The model under review builds one solid part; all positions refer to its coordinate system, in mm. A direction names the side the tool comes from. Coordinates: 2 decimals unless noted, no trailing zeros. Write each loop counter-clockwise with the first axis right and the second up, starting at its lowest first coordinate (ties: lowest second). Pieces come first, ordered by that corner, then holes. Notation, with made-up numbers: (88.5, -5) - (133.5, -5) arc R15 cw to (133.5, 18) - close; hole circle Ø10 at (-21.5, 53). An arc over 180 degrees is marked (long way). Use one line per item in the form item = value. Start each with the question number.
```python
from build123d import *

# Parameters (mm, degrees)
SKETCH_W        = 95
SKETCH_H        = 27
PAD_DEPTH       = 2
SKETCH001_R     = 1.3
POCKET_DEPTH    = 2
FILLET_R        = 3
SKETCH002_W     = 9.2
SKETCH002_H     = 11.4
POCKET001_DEPTH = 2
SKETCH003_W     = 13.2
SKETCH003_H     = 11.4
SKETCH003_W_2   = 18.2
SKETCH003_H_2   = 11.5
POCKET002_DEPTH = 2


with BuildPart() as part:
    # Sketch → Pad (new body)
    with BuildSketch(Plane.XY):
        Rectangle(SKETCH_W, SKETCH_H)
    extrude(amount=PAD_DEPTH)

    # Sketch001 (on Face6 of Pad) → Pocket (cut)
    with BuildSketch(Plane.XY.offset(2)):
        with Locations((-44.5, 10.5)):
            Circle(SKETCH001_R)
        with Locations((44.5, 10.5)):
            Circle(SKETCH001_R)
        with Locations((44.5, -10.5)):
            Circle(SKETCH001_R)
        with Locations((-44.5, -10.5)):
            Circle(SKETCH001_R)
    extrude(amount=-POCKET_DEPTH, mode=Mode.SUBTRACT)

    # Fillet
    fillet_edges = [part.edges().sort_by_distance(p)[0] for p in [
        (-47.5, -13.5, 1),
        (47.5, -13.5, 1),
        (47.5, 13.5, 1),
        (-47.5, 13.5, 1),
    ]]
    fillet(fillet_edges, radius=FILLET_R)

    # Sketch002 (on Face5 of Fillet) → Pocket001 (cut)
    with BuildSketch(Plane.XY.offset(2)):
        with Locations((31.3, 1.1)):
            Rectangle(SKETCH002_W, SKETCH002_H)
    extrude(amount=-POCKET001_DEPTH, mode=Mode.SUBTRACT)

    # Sketch003 (on Face5 of Pocket001) → Pocket002 (cut)
    with BuildSketch(Plane.XY.offset(2)):
        with Locations((4, 1.1)):
            Rectangle(SKETCH003_W, SKETCH003_H)
        with Locations((-26.2, 1.15)):
            Rectangle(SKETCH003_W_2, SKETCH003_H_2)
    extrude(amount=-POCKET002_DEPTH, mode=Mode.SUBTRACT)


solid = part.part
```
1. The part is to be moulded in two halves that separate along X. For faces 1 (the cylindrical face through (46.6, 12.64, 1.01)), 2 (the cylindrical face through (-46.64, 12.6, 1.01)), 3 (the flat face through (4, -4.6, 1)), say which applies: released by +X, released by -X, zero draft, split by the parting line, or undercut.
2. For P1, Ø2.5, axis at x = -44.5, y = -10.5, coming from the -Z side, flat-tipped, find the tip position at first contact; note if it passes through.
3. For L1, parallel to Y at x = -44.5, z = 1.4; L2, parallel to X at y = 1, z = 1.1; L3, parallel to Y at x = -19.5, z = 0.2, list the stretches that pass through material, from the lowest coordinate up.
4. Take a section at A-A (x = 8.5). State the section outline as (y, z) points.
5. Take a section at B-B (z = 1.05). State the section outline as (x, y) points, plus the area to 3 significant figures.
6. Take a section at C-C (y = -0.5). State the section outline as (x, z) points, plus the area to 3 significant figures.
7. For faces 4 (the flat face through (-1, -6, 0)), 5 (the flat face through (-2.6, 1, 1)), list the 3-axis set-ups (+Z, -Z, +X, -X, +Y, -Y) from which the entire face can be reached by the end or side of a thin tool; tool diameter is ignored.
Returned:
q1.face_1 = released by +X
q1.face_2 = released by -X
q1.face_3 = undercut
q2.P1 = through
q3.L1 = -13.5 to -11.8, -9.2 to 9.2, 11.8 to 13.5
q3.L2 = -47.5 to -35.3, -17.1 to -2.6, 10.6 to 26.7, 35.9 to 47.5
q3.L3 = -13.5 to -4.6, 6.9 to 13.5
q4.outline = (-13.5, 0) - (-4.6, 0) - (-4.6, 2) - (-13.5, 2) - close; (6.8, 0) - (13.5, 0) - (13.5, 2) - (6.8, 2) - close
q5.outline = (-47.5, -10.5) arc R3 ccw to (-44.5, -13.5) - (44.5, -13.5) arc R3 ccw to (47.5, -10.5) - (47.5, 10.5) arc R3 ccw to (44.5, 13.5) - (-44.5, 13.5) arc R3 ccw to (-47.5, 10.5) - close; hole circle Ø2.6 at (-44.5, -10.5); hole circle Ø2.6 at (-44.5, 10.5); hole (-35.3, -4.6) - (-17.1, -4.6) - (-17.1, 6.9) - (-35.3, 6.9) - close; hole (-2.6, -4.6) - (10.6, -4.6) - (10.6, 6.8) - (-2.6, 6.8) - close; hole (26.7, -4.6) - (35.9, -4.6) - (35.9, 6.8) - (26.7, 6.8) - close; hole circle Ø2.6 at (44.5, -10.5); hole circle Ø2.6 at (44.5, 10.5)
q5.area = 2,070 mm²
q6.outline = (-47.5, 0) - (-35.3, 0) - (-35.3, 2) - (-47.5, 2) - close; (-17.1, 0) - (-2.6, 0) - (-2.6, 2) - (-17.1, 2) - close; (10.6, 0) - (26.7, 0) - (26.7, 2) - (10.6, 2) - close; (35.9, 0) - (47.5, 0) - (47.5, 2) - (35.9, 2) - close
q6.area = 109 mm²
q7.face_4 = -Z, +X, -X, +Y, -Y
q7.face_5 = +Z, -Z
